Job drawing, mm, ordinate dimensions from the low corner. One solid piece. A direction names the side the tool comes from. Round coordinates to 2 decimals unless told otherwise and drop trailing zeros. Loops run counter-clockwise (first coordinate to the right, second up) from the corner with the lowest first, then second, coordinate; pieces in that order, holes last.
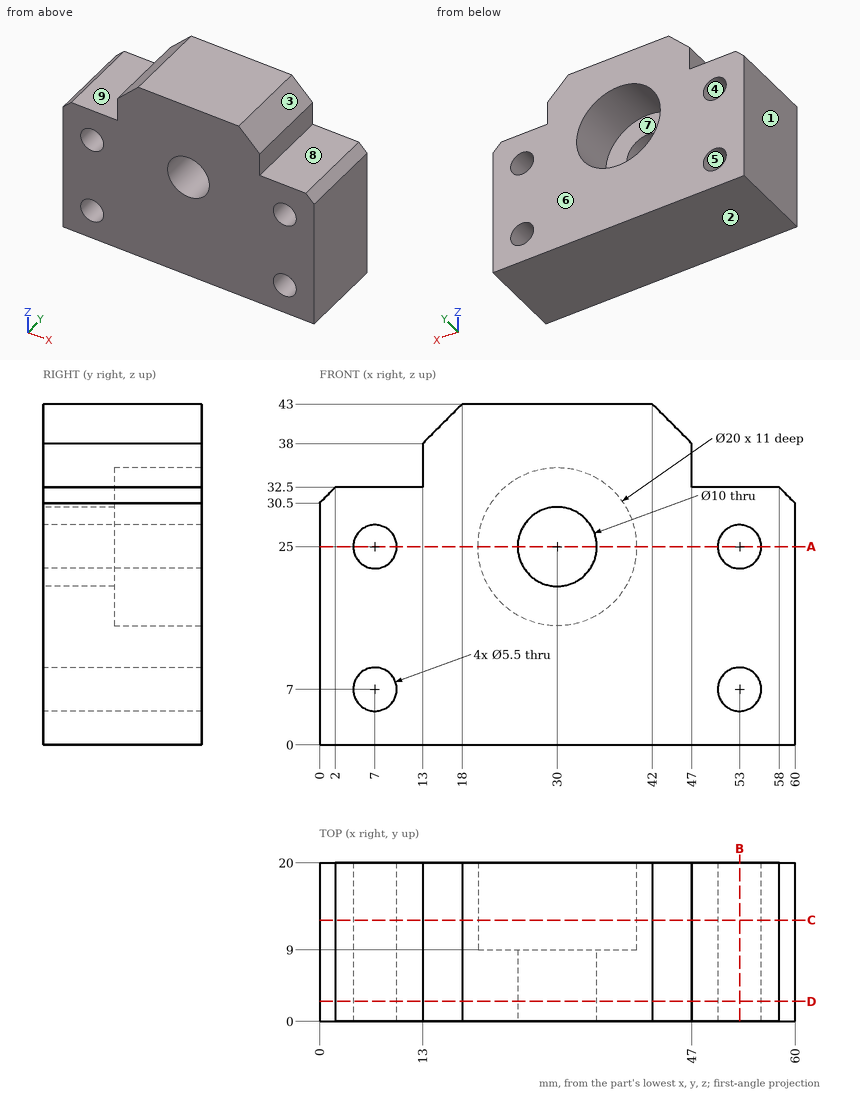
1) Slice it at C-C, the plane y = 12.75. Give the cut face in (x, z).
Values:
outline: (0, 0) - (60, 0) - (60, 30.5) - (58, 32.5) - (47, 32.5) - (47, 38) - (42, 43) - (18, 43) - (13, 38) - (13, 32.5) - (2, 32.5) - (0, 30.5) - close; hole circle Ø5.5 at (7, 7); hole circle Ø5.5 at (7, 25); hole circle Ø20 at (30, 25); hole circle Ø5.5 at (53, 7); hole circle Ø5.5 at (53, 25)
2) Tool access for the marked faces 5, 6, 7, 8 and 9: list every direction of +Z, -Z, +X, -X, +Y, -Y with a clear straight run to the whole face (end or side of a thin tool).
Values:
face 5: +Y, -Y
face 6: +Z, -Z, +X, -X, +Y
face 7: +Y
face 8: +Z, +X, +Y, -Y
face 9: +Z, -X, +Y, -Y
3) Slice it at A-A, the plane z = 25. Give the cut face in (x, y), then the cut area to 3 significant figures.
Values:
outline: (0, 0) - (4.25, 0) - (4.25, 20) - (0, 20) - close; (9.75, 0) - (25, 0) - (25, 9) - (20, 9) - (20, 20) - (9.75, 20) - close; (35, 0) - (50.25, 0) - (50.25, 20) - (40, 20) - (40, 9) - (35, 9) - close; (55.75, 0) - (60, 0) - (60, 20) - (55.75, 20) - close
area: 670 mm2
4) Wall check: line 1 along Z through (x, y) = (30, 16.5); line 2 along Z through (x, y) = (53, 7.25); line 3 along Z through (x, y) = (9, 3). Give the ranges that are in metal, low to high.
Values:
line 1: z = 0 to 15, 35 to 43
line 2: z = 0 to 4.25, 9.75 to 22.25, 27.75 to 32.5
line 3: z = 0 to 5.11, 8.89 to 23.11, 26.89 to 32.5
5) Slice it at B-B, the plane x = 53. Give the cut face in (y, z).
Values:
outline: (0, 0) - (20, 0) - (20, 4.25) - (0, 4.25) - close; (0, 9.75) - (20, 9.75) - (20, 22.25) - (0, 22.25) - close; (0, 27.75) - (20, 27.75) - (20, 32.5) - (0, 32.5) - close
6) Slice it at D-D, the plane y = 2.5. Give the cut face in (x, z), then the cut area to 3 significant figures.
Values:
outline: (0, 0) - (60, 0) - (60, 30.5) - (58, 32.5) - (47, 32.5) - (47, 38) - (42, 43) - (18, 43) - (13, 38) - (13, 32.5) - (2, 32.5) - (0, 30.5) - close; hole circle Ø5.5 at (7, 7); hole circle Ø5.5 at (7, 25); hole circle Ø10 at (30, 25); hole circle Ø5.5 at (53, 7); hole circle Ø5.5 at (53, 25)
area: 2,100 mm2
7) Drop flat-ended pins along their axis: pin 1 Ø3.5 at (x, y) = (5.5, 12.5) entering from +Z; pin 2 Ø9 at (x, z) = (7, 25) entering from +Y; pin 3 Ø6 at (x, z) = (30, 25) entering from -Y; pin 4 Ø6 at (y, z) = (5.5, 34) entering from +X. Give the stop position or say it passes through.
Values:
pin 1: stops at z = 32.5
pin 2: stops at y = 20
pin 3: passes through
pin 4: stops at x = 59.5
8) Mould opens along Z. For the marked faces 1, 2, 3 and 4 say: released by +Z, released by -Z, zero draft, split by the parting line, or undercut.
Values:
face 1: zero draft
face 2: released by -Z
face 3: released by +Z
face 4: undercut
